from build123d import *

# Parameters (mm, degrees)
BOSS_EXTRUDE1_DEPTH  = 6.35
M3_CLEARANCE_HOLE3_D = 2
M3_CLEARANCE_HOLE2_D = 2.5


with BuildPart() as part:
    # Sketch7 → Boss-Extrude1 (new body)
    with BuildSketch(Plane.XY):
        with BuildLine():
            Line((-119.9, -122.4), (119.9, -122.4))
            ThreePointArc((119.9, -122.4), (121.667766953, -123.132233047), (122.4, -124.9))
            Line((122.4, -124.9), (122.4, -149.9))
            ThreePointArc((122.4, -149.9), (123.132233047, -151.667766953), (124.9, -152.4))
            Line((124.9, -152.4), (149.9, -152.4))
            ThreePointArc((149.9, -152.4), (151.667766953, -151.667766953), (152.4, -149.9))
            Line((152.4, -149.9), (152.4, -102.186961883))
            Line((152.4, -102.186961883), (152.4, 120.74319893))
            Line((152.4, 120.74319893), (152.4, 149.9))
            ThreePointArc((152.4, 149.9), (151.667766953, 151.667766953), (149.9, 152.4))
            Line((149.9, 152.4), (124.9, 152.4))
            ThreePointArc((124.9, 152.4), (123.132233047, 151.667766953), (122.4, 149.9))
            Line((122.4, 149.9), (122.4, 124.9))
            ThreePointArc((122.4, 124.9), (121.667766953, 123.132233047), (119.9, 122.4))
            Line((119.9, 122.4), (-119.9, 122.4))
            ThreePointArc((-119.9, 122.4), (-121.667766953, 123.132233047), (-122.4, 124.9))
            Line((-122.4, 124.9), (-122.4, 149.9))
            ThreePointArc((-122.4, 149.9), (-123.132233047, 151.667766953), (-124.9, 152.4))
            Line((-124.9, 152.4), (-149.9, 152.4))
            ThreePointArc((-149.9, 152.4), (-151.667766953, 151.667766953), (-152.4, 149.9))
            Line((-152.4, 149.9), (-152.4, 102.186961883))
            Line((-152.4, 102.186961883), (-152.4, -120.74319893))
            Line((-152.4, -120.74319893), (-152.4, -149.9))
            ThreePointArc((-152.4, -149.9), (-151.667766953, -151.667766953), (-149.9, -152.4))
            Line((-149.9, -152.4), (-124.9, -152.4))
            ThreePointArc((-124.9, -152.4), (-123.132233047, -151.667766953), (-122.4, -149.9))
            Line((-122.4, -149.9), (-122.4, -124.9))
            ThreePointArc((-122.4, -124.9), (-121.667766953, -123.132233047), (-119.9, -122.4))
        make_face()
        with BuildLine():
            Line((-119.9, -92.4), (119.9, -92.4))
            ThreePointArc((119.9, -92.4), (121.667766953, -91.667766953), (122.4, -89.9))
            Line((122.4, -89.9), (122.4, 89.9))
            ThreePointArc((122.4, 89.9), (121.667766953, 91.667766953), (119.9, 92.4))
            Line((119.9, 92.4), (-119.9, 92.4))
            ThreePointArc((-119.9, 92.4), (-121.667766953, 91.667766953), (-122.4, 89.9))
            Line((-122.4, 89.9), (-122.4, -89.9))
            ThreePointArc((-122.4, -89.9), (-121.667766953, -91.667766953), (-119.9, -92.4))
        make_face(mode=Mode.SUBTRACT)
    extrude(amount=BOSS_EXTRUDE1_DEPTH)

    # M3 Clearance Hole3 (through all)
    with Locations(Plane.XY.offset(6.35)):
        with Locations((-137.4, 107.4), (-137.4, -107.4), (137.4, -107.4), (137.4, 107.4)):
            Hole(M3_CLEARANCE_HOLE3_D / 2)

    # M3 Clearance Hole2 (through all)
    with Locations(Plane.XY.offset(6.35)):
        with Locations((-137.4, 137.4), (137.4, 137.4), (137.4, -137.4), (-137.4, -137.4)):
            Hole(M3_CLEARANCE_HOLE2_D / 2)


solid = part.part
Verification items for the finished model (mm, model axes). Give positions to 0.01 mm unless a question says otherwise; leave off trailing zeros. Order: outer loops, then holes, each group sorted by start corner. A loop starts at its lowest first (then second) coordinate and runs counter-clockwise, first axis right, second up. Notation, with made-up numbers: M 79,38.25 L 108,38.25 A33 ccw 108,71.25 Z; hole C 27,19 d1. An arc over 180 degrees is marked long. Answer as a JSON object with one key per item and string values. Group by question number.
1) Depth check by flat-ended pin: pin 1 Ø1.6 at (x, y) = (137.4, 107.4) entering from -Z; pin 2 Ø3 at (x, z) = (28, 2) entering from +Y; pin 3 Ø3 at (x, z) = (43, 2.5) entering from -Y. Enter the tip coordinate at first touch or a pass-through.
2) Cross-section at C-C (z = 2.75). Give the number of separate pieces and of enclosed holes in the cut face, then the cut area to 3 significant figures.
3) Cross-section at A-A (y = -46.5). Enter the section's corners in (x, z).
4) Scan lines: line 1 along Y through (x, z) = (-137.4, 3.5); line 2 along X through (y, z) = (-107.4, 2.25); line 3 along X through (y, z) = (137.4, 3.75). Record each from-to range of solid material in increasing order. Write a range as [from, to].
5) Cross-section at B-B (x = -70.5). Enter the section's corners in (y, z), then the cut area to 3 significant figures.
Result sheet:
{
 "1": {"pin 1": "passes through", "pin 2": "stops at y = 122.4", "pin 3": "stops at y = -122.4"},
 "2": {"separate pieces": "1", "enclosed holes": "9", "area": "32,900 mm2"},
 "3": {"outline": "M -152.4,0 L -122.4,0 L -122.4,6.35 L -152.4,6.35 Z; M 122.4,0 L 152.4,0 L 152.4,6.35 L 122.4,6.35 Z"},
 "4": {"line 1": "y = [-152.4, -138.65], [-136.15, -108.4], [-106.4, 106.4], [108.4, 136.15], [138.65, 152.4]", "line 2": "x = [-152.4, -138.4], [-136.4, 136.4], [138.4, 152.4]", "line 3": "x = [-152.4, -138.65], [-136.15, -122.4], [122.4, 136.15], [138.65, 152.4]"},
 "5": {"outline": "M -122.4,0 L -92.4,0 L -92.4,6.35 L -122.4,6.35 Z; M 92.4,0 L 122.4,0 L 122.4,6.35 L 92.4,6.35 Z", "area": "381 mm2"}
}
